Part model, mm, in its own coordinate system. Face numbers are marked on the shaded views. A direction names the side the tool comes from. Coordinates: 2 decimals unless noted, no trailing zeros. Loops run counter-clockwise (first coordinate to the right, second up) from the corner with the lowest first, then second, coordinate; pieces in that order, holes last. Notation, with made-up numbers: (-28, -1) - (22, -1) arc R26 ccw to (22, 32) - close; hole circle Ø2 at (12.25, -14.75). An arc over 180 degrees is marked (long way). Use a Markdown table: item, result. Add a question column.
1. Band-saw the part on C-C, the plane z = 14. Give the cut face in (x, y) (3 decimals).
2. Band-saw the part on A-A, the plane z = 2.5. Count the separate pieces of the cut face and the enclosed holes in it, plus the area to 3 significant figures.
3. Band-saw the part on B-B, the plane y = 47. Give the cut face in (x, z).
4. Drop flat-ended pins along their axis: pin 1 (1.2 mm diameter, centred on y = 41, z = -15, fed in from -X); pin 2 (5 mm diameter, centred on x = -52.5, z = -7.5, fed in from +Y) (3 decimals); pin 3 (5 mm diameter, centred on x = 54.5, z = 2, fed in from +Y) (3 decimals); pin 4 (10 mm diameter, centred on x = 40, y = 4.5, fed in from +Z). Give the stop position or say it passes through.
5. Wall check: probe 1 along X at (y, z) = (-16, -4); probe 2 along Y at (x, z) = (11, 14) (3 decimals); probe 3 along X at (y, z) = (19, 8.5) (3 decimals). Give the ranges that are in metal, low to high. Write a range as [from, to].
6. Pull direction Y, two halves, no side cores. Call the marked faces 4, 5 and 6: pulls with the +Y half, pulls with the -Y half, needs draft (parallel to the pull), parting line crosses it, or undercut.
7. Band-saw the part on D-D, the plane x = -14. Give the cut face in (y, z) (3 decimals).
8. 3-axis set-ups, long thin cutter, end or side, ignore diameter. For the marked faces 1, 2 and 3: which of +Z, -Z, +X, -X, +Y, -Y reach the whole face in a straight line?
from build123d import *

# Parameters (mm, degrees)
BOSS_EXTRUDE1_DEPTH = 17.5
CHAMFER1_SIZE       = 30
SKETCH6_W           = 5.15
SKETCH6_H           = 25.15
CUT_EXTRUDE2_DEPTH  = 4
SKETCH7_W           = 3
SKETCH7_H           = 20
CUT_EXTRUDE3_DEPTH  = 10
SKETCH8_W           = 5
SKETCH8_H           = 25
SKETCH8_W_2         = 2
SKETCH8_H_2         = 18
BOSS_EXTRUDE2_DEPTH = 3.5
CHAMFER2_SIZE       = 4
CHAMFER3_SIZE       = 2


# Some blends are built 0.0001 mm under size
with BuildPart() as part:
    # Sketch1 → Boss-Extrude1 (new, symmetric)
    with BuildSketch(Plane.XY):
        Polygon((55.75, -26.875), (55.75, -22.875), (51.25, -22.875), (51.25, -19.875), (55.75, -19.875), (55.75, 26.875), (-55.75, 26.875), (-55.75, -19.875), (-51.25, -19.875), (-51.25, -22.875), (-55.75, -22.875), (-55.75, -26.875), (-59.75, -26.875), (-59.75, 30.875), (59.75, 30.875), (59.75, -26.875), align=None)
    extrude(amount=BOSS_EXTRUDE1_DEPTH, both=True)

    # Chamfer1
    chamfer1_edges = [part.edges().sort_by_distance(p)[0] for p in [
        (-59.75, 30.875, 0),
        (59.75, 30.875, 0),
        (55.75, 26.875, 0),
        (-55.75, 26.875, 0),
    ]]
    chamfer(chamfer1_edges, length=CHAMFER1_SIZE)

    # Sketch6 → Cut-Extrude2 (cut)
    with BuildSketch(Plane(origin=(0, 30.875, 0), x_dir=(1, 0, 0), z_dir=(0, 1, 0))):
        Rectangle(SKETCH6_W, SKETCH6_H)
    extrude(amount=-CUT_EXTRUDE2_DEPTH, mode=Mode.SUBTRACT)

    # Sketch7 → Cut-Extrude3 (cut)
    with BuildSketch(Plane(origin=(0, 30.875, 0), x_dir=(1, 0, 0), z_dir=(0, 1, 0))):
        with Locations((10.4, 0)):
            Rectangle(SKETCH7_W, SKETCH7_H)
        with Locations((-10.4, 0)):
            Rectangle(SKETCH7_W, SKETCH7_H)
    extrude(amount=-CUT_EXTRUDE3_DEPTH, mode=Mode.SUBTRACT)

    # Sketch8 → Boss-Extrude2 (add)
    with BuildSketch(Plane.XY.offset(-17.5)):
        with Locations((-23.25, 39.375)):
            Rectangle(SKETCH8_W, SKETCH8_H)
        with Locations((-23.25, 41.375)):
            Rectangle(SKETCH8_W_2, SKETCH8_H_2, mode=Mode.SUBTRACT)
    extrude(amount=BOSS_EXTRUDE2_DEPTH)

    # Chamfer2
    chamfer2_edges = [part.edges().sort_by_distance(p)[0] for p in [
        (-20.75, 30.875, -15.75),
        (-25.75, 30.875, -15.75),
    ]]
    chamfer(chamfer2_edges, length=CHAMFER2_SIZE - 0.0001)  # a hair under: the kernel refuses the full size

    # Chamfer3
    # the kernel refuses this chamfer: 2 mm, written as the material it adds along each edge
    with BuildSketch(Plane(origin=(-11.606734024, 30.875, -14), x_dir=(0, 0.9996219169112968, -0.02749587661058651), z_dir=(-1, 0, 0))) as chamfer3_piece_1_section:
        Polygon((CHAMFER3_SIZE * 0.999621916911, -CHAMFER3_SIZE * 0.0274958766106), (-CHAMFER3_SIZE * 0.0274958766106, -CHAMFER3_SIZE * 0.999621916911), (0, 0), align=None)
    chamfer3_piece_1 = extrude(amount=23.286531952, mode=Mode.PRIVATE)
    chamfer3_piece_1 = split(chamfer3_piece_1, bisect_by=Plane(origin=(-22.25, 32.567452132, -13.881504022), z_dir=(1, 0, 0)), keep=Keep.TOP, mode=Mode.PRIVATE)
    chamfer3_piece_1 = split(chamfer3_piece_1, bisect_by=Plane(origin=(-19.394414099, 33.519314099, -13.881504022), z_dir=(-0.7071067811865476, -0.7071067811865476, 0)), keep=Keep.TOP, mode=Mode.PRIVATE)
    chamfer3_piece_1 = split(chamfer3_piece_1, bisect_by=Plane(origin=(-20.346276066, 32.375, -13.881504022), z_dir=(0, 1, 0)), keep=Keep.TOP, mode=Mode.PRIVATE)
    add(chamfer3_piece_1)
    with BuildSketch(Plane(origin=(-11.606734024, 30.875, -14), x_dir=(0, 0.9996219169112968, -0.02749587661058651), z_dir=(-1, 0, 0))) as chamfer3_piece_2_section:
        Polygon((CHAMFER3_SIZE * 0.999621916911, -CHAMFER3_SIZE * 0.0274958766106), (-CHAMFER3_SIZE * 0.0274958766106, -CHAMFER3_SIZE * 0.999621916911), (0, 0), align=None)
    chamfer3_piece_2 = extrude(amount=23.286531952, mode=Mode.PRIVATE)
    chamfer3_piece_2 = split(chamfer3_piece_2, bisect_by=Plane(origin=(-22.25, 31.41379866, -13.276536182), z_dir=(1, 0, 0)), keep=Keep.TOP, mode=Mode.PRIVATE)
    chamfer3_piece_2 = split(chamfer3_piece_2, bisect_by=Plane(origin=(-18.529173995, 32.654073995, -13.276536182), z_dir=(-0.7071067811865476, -0.7071067811865476, 0)), keep=Keep.TOP, mode=Mode.PRIVATE)
    chamfer3_piece_2 = split(chamfer3_piece_2, bisect_by=Plane(origin=(-19.76944933, 32.375, -13.276536182), z_dir=(0, -1, 0)), keep=Keep.TOP, mode=Mode.PRIVATE)
    add(chamfer3_piece_2)
    with BuildSketch(Plane(origin=(-11.606734024, 30.875, -14), x_dir=(0, 0.9996219169112968, -0.02749587661058651), z_dir=(-1, 0, 0))) as chamfer3_piece_3_section:
        Polygon((CHAMFER3_SIZE * 0.999621916911, -CHAMFER3_SIZE * 0.0274958766106), (-CHAMFER3_SIZE * 0.0274958766106, -CHAMFER3_SIZE * 0.999621916911), (0, 0), align=None)
    chamfer3_piece_3 = extrude(amount=23.286531952, mode=Mode.PRIVATE)
    chamfer3_piece_3 = split(chamfer3_piece_3, bisect_by=Plane(origin=(-22.25, 31.449972825, -13.29608178), z_dir=(-1, 0, 0)), keep=Keep.TOP, mode=Mode.PRIVATE)
    chamfer3_piece_3 = split(chamfer3_piece_3, bisect_by=Plane(origin=(-23.25, 32.375, -13.29608178), z_dir=(0, -1, 0)), keep=Keep.TOP, mode=Mode.PRIVATE)
    chamfer3_piece_3 = split(chamfer3_piece_3, bisect_by=Plane(origin=(-24.25, 31.449972825, -13.29608178), z_dir=(1, 0, 0)), keep=Keep.TOP, mode=Mode.PRIVATE)
    add(chamfer3_piece_3)
    with BuildSketch(Plane(origin=(-11.606734024, 30.875, -14), x_dir=(0, 0.9996219169112968, -0.02749587661058651), z_dir=(-1, 0, 0))) as chamfer3_piece_4_section:
        Polygon((CHAMFER3_SIZE * 0.999621916911, -CHAMFER3_SIZE * 0.0274958766106), (-CHAMFER3_SIZE * 0.0274958766106, -CHAMFER3_SIZE * 0.999621916911), (0, 0), align=None)
    chamfer3_piece_4 = extrude(amount=23.286531952, mode=Mode.PRIVATE)
    chamfer3_piece_4 = split(chamfer3_piece_4, bisect_by=Plane(origin=(-27.105585901, 33.519314099, -13.881504022), z_dir=(0.7071067811865472, -0.7071067811865478, 0)), keep=Keep.TOP, mode=Mode.PRIVATE)
    chamfer3_piece_4 = split(chamfer3_piece_4, bisect_by=Plane(origin=(-26.153723934, 32.375, -13.881504022), z_dir=(0, 1, 0)), keep=Keep.TOP, mode=Mode.PRIVATE)
    chamfer3_piece_4 = split(chamfer3_piece_4, bisect_by=Plane(origin=(-24.25, 32.567452132, -13.881504022), z_dir=(-1, 0, 0)), keep=Keep.TOP, mode=Mode.PRIVATE)
    add(chamfer3_piece_4)
    with BuildSketch(Plane(origin=(-11.606734024, 30.875, -14), x_dir=(0, 0.9996219169112968, -0.02749587661058651), z_dir=(-1, 0, 0))) as chamfer3_piece_5_section:
        Polygon((CHAMFER3_SIZE * 0.999621916911, -CHAMFER3_SIZE * 0.0274958766106), (-CHAMFER3_SIZE * 0.0274958766106, -CHAMFER3_SIZE * 0.999621916911), (0, 0), align=None)
    chamfer3_piece_5 = extrude(amount=23.286531952, mode=Mode.PRIVATE)
    chamfer3_piece_5 = split(chamfer3_piece_5, bisect_by=Plane(origin=(-27.970826005, 32.654073995, -13.276536182), z_dir=(0.7071067811865472, -0.7071067811865478, 0)), keep=Keep.TOP, mode=Mode.PRIVATE)
    chamfer3_piece_5 = split(chamfer3_piece_5, bisect_by=Plane(origin=(-26.73055067, 32.375, -13.276536182), z_dir=(0, -1, 0)), keep=Keep.TOP, mode=Mode.PRIVATE)
    chamfer3_piece_5 = split(chamfer3_piece_5, bisect_by=Plane(origin=(-24.25, 31.41379866, -13.276536182), z_dir=(-1, 0, 0)), keep=Keep.TOP, mode=Mode.PRIVATE)
    add(chamfer3_piece_5)


solid = part.part
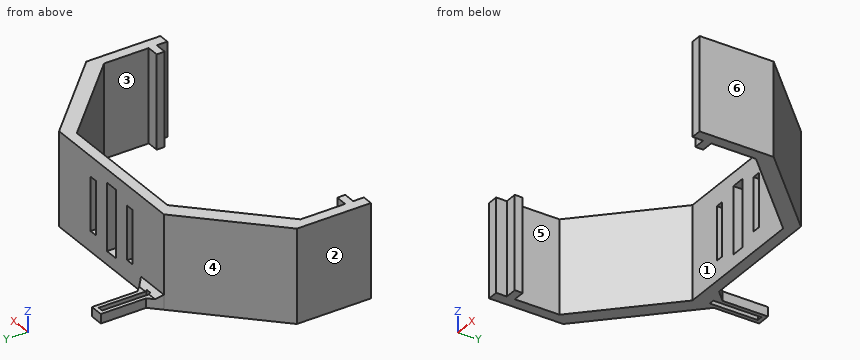
Geometry check:
| question | item | result |
|---|---|---|
| 1 | outline | (-59.75, -26.875) - (-55.75, -26.875) - (-55.75, -22.875) - (-51.25, -22.875) - (-51.25, -19.875) - (-55.75, -19.875) - (-55.75, -3.125) - (-25.75, 26.875) - (25.75, 26.875) - (55.75, -3.125) - (55.75, -19.875) - (51.25, -19.875) - (51.25, -22.875) - (55.75, -22.875) - (55.75, -26.875) - (59.75, -26.875) - (59.75, 0.875) - (29.75, 30.875) - (-29.75, 30.875) - (-59.75, 0.875) - close |
| 2 | separate pieces | 4 |
| 2 | enclosed holes | 0 |
| 2 | area | 890 mm^2 |
| 3 | outline | (-25.75, -17.5) - (-24.25, -17.5) - (-24.25, -14) - (-25.75, -14) - close; (-22.25, -17.5) - (-20.75, -17.5) - (-20.75, -14) - (-22.25, -14) - close |
| 4 | pin 1 | stops at x = -25.75 |
| 4 | pin 2 | stops at y = 10.625 |
| 4 | pin 3 | stops at y = 8.625 |
| 4 | pin 4 | passes through |
| 5 | probe 1 | x = [-59.75, -55.75], [55.75, 59.75] |
| 5 | probe 2 | y = [26.875, 30.875] |
| 5 | probe 3 | x = [-41.625, -33.625], [33.625, 41.625] |
| 6 | face 4 | pulls with the +Y half |
| 6 | face 5 | undercut |
| 6 | face 6 | needs draft |
| 7 | outline | (26.875, -17.5) - (30.875, -17.5) - (30.875, 17.5) - (26.875, 17.5) - close |
| 8 | face 1 | +Z, -Z, -Y |
| 8 | face 2 | +Z, -Z, -X, +Y, -Y |
| 8 | face 3 | +Z, -Z |
